Source: CAD feature listing. Evaluate the final solid. Frame: model axes, mm. Face numbers are marked on the shaded views. A direction names the side the tool comes from. Round coordinates to 2 decimals unless told otherwise and drop trailing zeros. Loops run counter-clockwise (first coordinate to the right, second up) from the corner with the lowest first, then second, coordinate; pieces in that order, holes last. Notation, with made-up numbers: (63.5, 84.5) - (97.5, 84.5) arc R15 cw to (97.5, 100.5) - close; hole circle Ø2 at (4.5, 4). An arc over 180 degrees is marked (long way). One line per question, with ' | ' between items. Start each with the question number.
1. Ray query, line 1 (X direction, y = 3.5, z = 0) (3 decimals); line 2 (X direction, y = 1.2, z = 0); line 3 (Z direction, x = 14, y = 3.25) (3 decimals). Return the intervals inside material, ascending.
2. Cut plane A-A (x = -14). Return loops of the section in (y, z) (3 decimals), then the cut area to 3 significant figures.
3. Pin query (flat end, axial travel): pin 1 (3 mm diameter, centred on x = -14, z = -6.5, fed in from +Y); pin 2 (1.5 mm diameter, centred on y = 8, z = 1.5, fed in from +X); pin 3 (3 mm diameter, centred on x = 0.5, z = 16, fed in from +Y). Return the tip coordinate at first contact, or that it passes through.
4. Cut plane B-B (z = 14). Return loops of the section in (x, y) (3 decimals), then the cut area to 3 significant figures.
5. Access query for the marked faces 4, 5, 6 and 7. Directions: +Z, -Z, +X, -X, +Y, -Y. A direction counts if a zero-diameter tool reaches every point of the face in a straight line with its end or side. Return the directions, or none.
6. Cut plane D-D (z = 0). State how many separate pieces and enclosed holes the cut face has, then the cut area to 3 significant figures.
7. Mould query, pull axis X, two halves, no side actions, for the marked faces 1, 2 and 3. Classes: pulls with the +X half, pulls with the -X half, needs draft (parallel to the pull), parting line crosses it, or undercut.
8. Cut plane C-C (y = 6.5). Return loops of the section in (x, z).
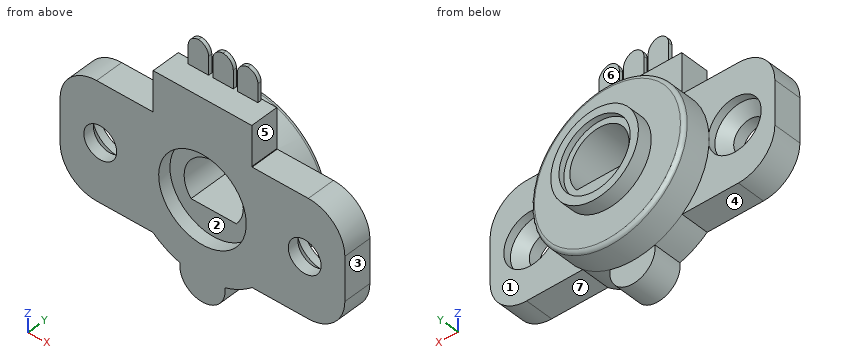
```python
from build123d import *

# Parameters (mm, degrees)
BOSS_EXTRUDE1_DEPTH = 3.9
SKETCH3_R           = 2.25
CUT_EXTRUDE1_DEPTH  = 25.091907
BOSS_EXTRUDE3_START = -3.9
SKETCH6_R           = 10.5
BOSS_EXTRUDE3_DEPTH = 7.8
SKETCH4_R           = 3.625
CUT_EXTRUDE2_DEPTH  = 2.4
BOSS_EXTRUDE4_START = -7.8
SKETCH7_R           = 6
BOSS_EXTRUDE4_DEPTH = 9.8
SKETCH8_R           = 4.875
CUT_EXTRUDE3_DEPTH  = 0.75
CUT_EXTRUDE4_DEPTH  = 26.438406
SKETCH10_R          = 6
CUT_EXTRUDE5_DEPTH  = 1.75
BOSS_EXTRUDE5_START = 3.2
SKETCH11_W          = 2.8
SKETCH11_H          = 4
BOSS_EXTRUDE5_DEPTH = 0.5
FILLET1_R           = 1.5
FILLET2_R           = 0.5


with BuildPart() as part:
    # Sketch2 → Boss-Extrude1 (new body)
    with BuildSketch(Plane(origin=(0, 0, 0), x_dir=(1, 0, 0), z_dir=(0, 1, 0))):
        with BuildLine():
            Line((-19.5, 3), (-19.5, -3))
            ThreePointArc((-19.5, -3), (-18.035534, -6.535534), (-14.5, -8))
            Line((-14.5, -8), (-6.75, -8))
            Line((-6.75, -8), (-6.75, -13.5))
            Line((-6.75, -13.5), (6.75, -13.5))
            Line((6.75, -13.5), (6.75, -8))
            Line((6.75, -8), (14.5, -8))
            ThreePointArc((14.5, -8), (18.035534, -6.535534), (19.5, -3))
            Line((19.5, -3), (19.5, 3))
            ThreePointArc((19.5, 3), (18.035534, 6.535534), (14.5, 8))
            Line((14.5, 8), (6.800735, 8))
            ThreePointArc((6.800735, 8), (5.037969, 9.21243), (3.066037, 10.042381))
            ThreePointArc((3.066037, 10.042381), (0, 13.6), (-3.066037, 10.042381))
            ThreePointArc((-3.066037, 10.042381), (-5.037969, 9.21243), (-6.800735, 8))
            Line((-6.800735, 8), (-14.5, 8))
            ThreePointArc((-14.5, 8), (-18.035534, 6.535534), (-19.5, 3))
        make_face()
    extrude(amount=BOSS_EXTRUDE1_DEPTH)

    # Sketch3 → Cut-Extrude1 (cut, through all)
    with BuildSketch(Plane(origin=(0, 3.9, 0), x_dir=(1, 0, 0), z_dir=(0, 1, 0))):
        with Locations(Location((-14, 0, 0), (0, 0, 270))):
            Circle(SKETCH3_R)
    cut_extrude1 = extrude(amount=-CUT_EXTRUDE1_DEPTH, mode=Mode.SUBTRACT)

    # Sketch6 → Boss-Extrude3 (add)
    with BuildSketch(Plane(origin=(0, 3.9, 0), x_dir=(1, 0, 0), z_dir=(0, 1, 0)).offset(BOSS_EXTRUDE3_START)):
        with Locations(Location((0, 0, 0), (0, 0, 73.022056))):
            Circle(SKETCH6_R)
    extrude(amount=BOSS_EXTRUDE3_DEPTH)

    # Sketch4 → Cut-Extrude2 (cut)
    with BuildSketch(Plane(origin=(0, 3.9, 0), x_dir=(1, 0, 0), z_dir=(0, 1, 0))):
        with Locations(Location((-14, 0, 0), (0, 0, 270))):
            Circle(SKETCH4_R)
    cut_extrude2 = extrude(amount=-CUT_EXTRUDE2_DEPTH, mode=Mode.SUBTRACT)

    # Sketch5 → Revolve1 (revolve)
    with BuildSketch(Plane.XY, mode=Mode.PRIVATE) as revolve1_sk:
        Polygon((-16.25, 1.5), (-17.625, 2.875), (-17.625, 1.5), align=None)
    revolve1 = revolve(revolve1_sk.sketch.rotate(Axis((-14, -999.202494, 0), (0, 1, 0)), 90), axis=Axis((-14, -999.202494, 0), (0, 1, 0)))

    # Mirror1: Cut-Extrude1, Cut-Extrude2, Revolve1 across plane
    add(cut_extrude1.mirror(Plane(origin=(0, 0, 0), x_dir=(0, 0, 1), z_dir=(1, 0, 0))), mode=Mode.SUBTRACT)
    add(cut_extrude2.mirror(Plane(origin=(0, 0, 0), x_dir=(0, 0, 1), z_dir=(1, 0, 0))), mode=Mode.SUBTRACT)
    add(revolve1.mirror(Plane(origin=(0, 0, 0), x_dir=(0, 0, 1), z_dir=(1, 0, 0))))

    # Sketch7 → Boss-Extrude4 (add)
    with BuildSketch(Plane(origin=(0, 7.8, 0), x_dir=(1, 0, 0), z_dir=(0, 1, 0)).offset(BOSS_EXTRUDE4_START)):
        with Locations(Location((0, 0, 0), (0, 0, 270))):
            Circle(SKETCH7_R)
    extrude(amount=BOSS_EXTRUDE4_DEPTH)

    # Sketch8 → Cut-Extrude3 (cut)
    with BuildSketch(Plane(origin=(0, 9.8, 0), x_dir=(1, 0, 0), z_dir=(0, 1, 0))):
        with Locations(Location((0, 0, 0), (0, 0, 270))):
            Circle(SKETCH8_R)
    extrude(amount=-CUT_EXTRUDE3_DEPTH, mode=Mode.SUBTRACT)

    # Sketch9 → Cut-Extrude4 (cut, through all)
    with BuildSketch(Plane(origin=(0, 9.05, 0), x_dir=(1, 0, 0), z_dir=(0, 1, 0))):
        with BuildLine():
            Line((-3.105238, 2.6), (3.105238, 2.6))
            ThreePointArc((3.105238, 2.6), (0, -4.05), (-3.105238, 2.6))
        make_face()
    extrude(amount=-CUT_EXTRUDE4_DEPTH, mode=Mode.SUBTRACT)

    # Sketch10 → Cut-Extrude5 (cut)
    with BuildSketch(Plane.XZ):
        with Locations(Location((0, 0, 0), (0, 0, 90))):
            Circle(SKETCH10_R)
    extrude(amount=-CUT_EXTRUDE5_DEPTH, mode=Mode.SUBTRACT)

    # Sketch11 → Boss-Extrude5 (add)
    with BuildSketch(Plane(origin=(0, 0, 0), x_dir=(1, 0, 0), z_dir=(0, 1, 0)).offset(BOSS_EXTRUDE5_START)):
        with Locations((-3.375, -15.5)):
            Rectangle(SKETCH11_W, SKETCH11_H)
        with Locations((0, -15.5)):
            Rectangle(SKETCH11_W, SKETCH11_H)
        with Locations((3.375, -15.5)):
            Rectangle(SKETCH11_W, SKETCH11_H)
    extrude(amount=BOSS_EXTRUDE5_DEPTH)

    # Fillet1
    # the kernel refuses this fillet: 1.5 mm, written as the material it takes off along each edge
    with BuildSketch(Plane(origin=(-4.775, -0.55, 17.5), x_dir=(0, 0, -1), z_dir=(0, 1, 0)), Plane(origin=(-1.4, -0.55, 17.5), x_dir=(0, 0, -1), z_dir=(0, 1, 0)), Plane(origin=(1.975, -0.55, 17.5), x_dir=(0, 0, -1), z_dir=(0, 1, 0))) as fillet1_piece_1:
        with BuildLine():
            CenterArc((FILLET1_R, -FILLET1_R), FILLET1_R, 90, 90)
            Line((0, -FILLET1_R), (0, 0))
            Line((0, 0), (FILLET1_R, 0))
        make_face()
    extrude(amount=8, mode=Mode.SUBTRACT)
    with BuildSketch(Plane(origin=(-1.975, -0.55, 17.5), x_dir=(0, 0, -1), z_dir=(0, 1, 0)), Plane(origin=(1.4, -0.55, 17.5), x_dir=(0, 0, -1), z_dir=(0, 1, 0)), Plane(origin=(4.775, -0.55, 17.5), x_dir=(0, 0, -1), z_dir=(0, 1, 0))) as fillet1_piece_2:
        with BuildLine():
            CenterArc((FILLET1_R, FILLET1_R), FILLET1_R, 180, 90)
            Line((0, FILLET1_R), (0, 0))
            Line((0, 0), (FILLET1_R, 0))
        make_face()
    extrude(amount=8, mode=Mode.SUBTRACT)

    # Fillet2
    fillet2_edges = [part.edges().sort_by_distance(p)[0] for p in [
        (-3.066037, 7.8, 10.042381),
    ]]
    fillet(fillet2_edges, radius=FILLET2_R)


solid = part.part
```
Answers follow:
1) line 1: x = -19.5 to -17.625, -10.375 to -4.05, 4.05 to 10.375, 17.625 to 19.5 | line 2: x = -19.5 to -16.25, -11.75 to -6, 6 to 11.75, 16.25 to 19.5 | line 3: z = -8 to -3.625, 3.625 to 8
2) outline: (0, -8) - (3.9, -8) - (3.9, -3.625) - (2.875, -3.625) - (1.5, -2.25) - (0, -2.25) - close; (0, 2.25) - (1.5, 2.25) - (2.875, 3.625) - (3.9, 3.625) - (3.9, 8) - (0, 8) - close | area: 40.1 mm2
3) pin 1: stops at y = 3.9 | pin 2: stops at x = 10.44 | pin 3: stops at y = 3.7
4) outline: (-4.775, 3.2) - (-1.975, 3.2) - (-1.975, 3.7) - (-4.775, 3.7) - close; (-1.4, 3.2) - (1.4, 3.2) - (1.4, 3.7) - (-1.4, 3.7) - close; (1.975, 3.2) - (4.775, 3.2) - (4.775, 3.7) - (1.975, 3.7) - close | area: 4.20 mm2
5) face 4: -Z, -X, +Y, -Y | face 5: +Z, +X, +Y, -Y | face 6: +Z, +X, -X, +Y | face 7: -Z, +X, +Y, -Y
6) separate pieces: 4 | enclosed holes: 0 | area: 126 mm2
7) face 1: needs draft | face 2: undercut | face 3: pulls with the +X half
8) outline: circle Ø21 at (0, 0); hole (-3.11, -2.6) - (3.11, -2.6) arc R4.05 ccw (long way) to start
